Build history of the part. All positions in model axes, mm. Face numbers are marked on the shaded views. Round coordinates to 2 decimals unless told otherwise and drop trailing zeros. Write each loop counter-clockwise with the first axis right and the second up, starting at its lowest first coordinate (ties: lowest second). Pieces come first, ordered by that corner, then holes. Notation, with made-up numbers: (22.5, -38.75) -> (65.5, -38.75) arc R33 ccw to (65.5, -8.75) -> close; hole circle Ø9 at (17, 71). An arc over 180 degrees is marked (long way). Answer in a Markdown table with one row per item.
```python
from build123d import *

# Parameters (mm, degrees)
SKETCH2_W           = 4.84
SKETCH2_H           = 1.78
BOSS_EXTRUDE1_DEPTH = 4.6
SKETCH3_R           = 0.22
CUT_EXTRUDE1_DEPTH  = 4.5
SKETCH5_R           = 0.1
BOSS_EXTRUDE2_DEPTH = 2.5


with BuildPart() as part:
    # Sketch2 → Boss-Extrude1 (new body)
    with BuildSketch(Plane(origin=(0, 0, 0), x_dir=(1, 0, 0), z_dir=(0, 1, 0))):
        with Locations((2.42, 0.89)):
            Rectangle(SKETCH2_W, SKETCH2_H)
    extrude(amount=BOSS_EXTRUDE1_DEPTH)

    # Sketch3 → Cut-Extrude1 (cut)
    with BuildSketch(Plane(origin=(0, 4.6, 0), x_dir=(1, 0, 0), z_dir=(0, 1, 0))):
        with Locations(Location((0.5, 1.48, 0), (0, 0, 270))):
            Circle(SKETCH3_R)
        with Locations(Location((1.14, 1.48, 0), (0, 0, 270))):
            Circle(SKETCH3_R)
        with Locations(Location((1.78, 1.48, 0), (0, 0, 270))):
            Circle(SKETCH3_R)
        with Locations(Location((2.42, 1.48, 0), (0, 0, 270))):
            Circle(SKETCH3_R)
        with Locations(Location((3.06, 1.48, 0), (0, 0, 270))):
            Circle(SKETCH3_R)
        with Locations(Location((3.7, 1.48, 0), (0, 0, 270))):
            Circle(SKETCH3_R)
        with Locations(Location((4.34, 1.48, 0), (0, 0, 270))):
            Circle(SKETCH3_R)
        with Locations(Location((0.5, 0.3, 0), (0, 0, 270))):
            Circle(SKETCH3_R)
        with Locations(Location((1.14, 0.3, 0), (0, 0, 270))):
            Circle(SKETCH3_R)
        with Locations(Location((1.78, 0.3, 0), (0, 0, 270))):
            Circle(SKETCH3_R)
        with Locations(Location((2.42, 0.3, 0), (0, 0, 270))):
            Circle(SKETCH3_R)
        with Locations(Location((3.06, 0.3, 0), (0, 0, 270))):
            Circle(SKETCH3_R)
        with Locations(Location((3.7, 0.3, 0), (0, 0, 270))):
            Circle(SKETCH3_R)
        with Locations(Location((4.34, 0.3, 0), (0, 0, 270))):
            Circle(SKETCH3_R)
    extrude(amount=-CUT_EXTRUDE1_DEPTH, mode=Mode.SUBTRACT)

    # Sketch5 → Boss-Extrude2 (add)
    with BuildSketch(Plane.XZ):
        with Locations(Location((0.5, -0.3, 0), (0, 0, 270))):
            Circle(SKETCH5_R)
        with Locations(Location((1.14, -0.3, 0), (0, 0, 270))):
            Circle(SKETCH5_R)
        with Locations(Location((1.78, -0.3, 0), (0, 0, 270))):
            Circle(SKETCH5_R)
        with Locations(Location((2.42, -0.3, 0), (0, 0, 270))):
            Circle(SKETCH5_R)
        with Locations(Location((3.06, -0.3, 0), (0, 0, 270))):
            Circle(SKETCH5_R)
        with Locations(Location((3.7, -0.3, 0), (0, 0, 270))):
            Circle(SKETCH5_R)
        with Locations(Location((4.34, -0.3, 0), (0, 0, 270))):
            Circle(SKETCH5_R)
        with Locations(Location((0.5, -1.48, 0), (0, 0, 270))):
            Circle(SKETCH5_R)
        with Locations(Location((1.14, -1.48, 0), (0, 0, 270))):
            Circle(SKETCH5_R)
        with Locations(Location((1.78, -1.48, 0), (0, 0, 270))):
            Circle(SKETCH5_R)
        with Locations(Location((2.42, -1.48, 0), (0, 0, 270))):
            Circle(SKETCH5_R)
        with Locations(Location((3.06, -1.48, 0), (0, 0, 270))):
            Circle(SKETCH5_R)
        with Locations(Location((3.7, -1.48, 0), (0, 0, 270))):
            Circle(SKETCH5_R)
        with Locations(Location((4.34, -1.48, 0), (0, 0, 270))):
            Circle(SKETCH5_R)
    extrude(amount=BOSS_EXTRUDE2_DEPTH)


solid = part.part
```
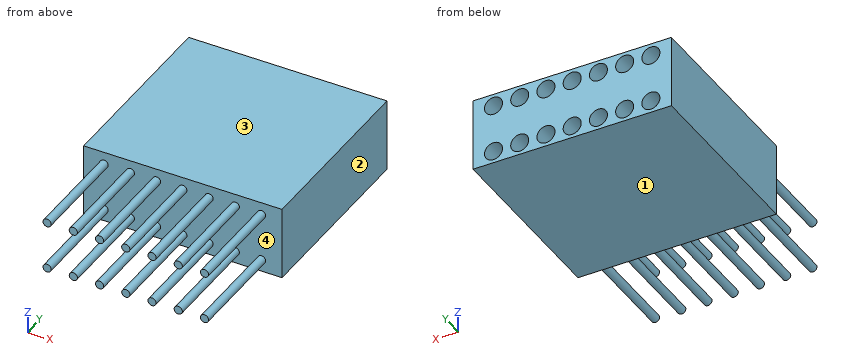
Q1. Wall check: line 1 (Y direction, x = 4, z = -0.45). Give the ranges that are in metal, low to high. Write a range as [from, to].
A:
| item | result |
|---|---|
| line 1 | [0, 4.6] |
Q2. Saw through at A-A on y = 2. State how many separate pieces and enclosed holes the cut face has, plus the area to 3 significant figures.
A:
| item | result |
|---|---|
| separate pieces | 1 |
| enclosed holes | 14 |
| area | 6.49 mm² |
Q3. Two-plate mould, pull along Z, no slides. Class the marked faces 1, 2, 3 and 4: released by +Z, released by -Z, zero draft, split by the parting line, or undercut.
A:
| item | result |
|---|---|
| face 1 | released by -Z |
| face 2 | zero draft |
| face 3 | released by +Z |
| face 4 | undercut |
Q4. Saw through at C-C on x = 0.5. Write the cut outline in (y, z).
A:
| item | result |
|---|---|
| outline | (-2.5, -1.58) -> (0, -1.58) -> (0, -1.78) -> (4.6, -1.78) -> (4.6, -1.7) -> (0.1, -1.7) -> (0.1, -1.26) -> (4.6, -1.26) -> (4.6, -0.52) -> (0.1, -0.52) -> (0.1, -0.08) -> (4.6, -0.08) -> (4.6, 0) -> (0, 0) -> (0, -0.2) -> (-2.5, -0.2) -> (-2.5, -0.4) -> (0, -0.4) -> (0, -1.38) -> (-2.5, -1.38) -> close |
Q5. Saw through at D-D on z = -0.85. Write the cut outline in (x, y).
A:
| item | result |
|---|---|
| outline | (0, 0) -> (4.84, 0) -> (4.84, 4.6) -> (0, 4.6) -> close |
